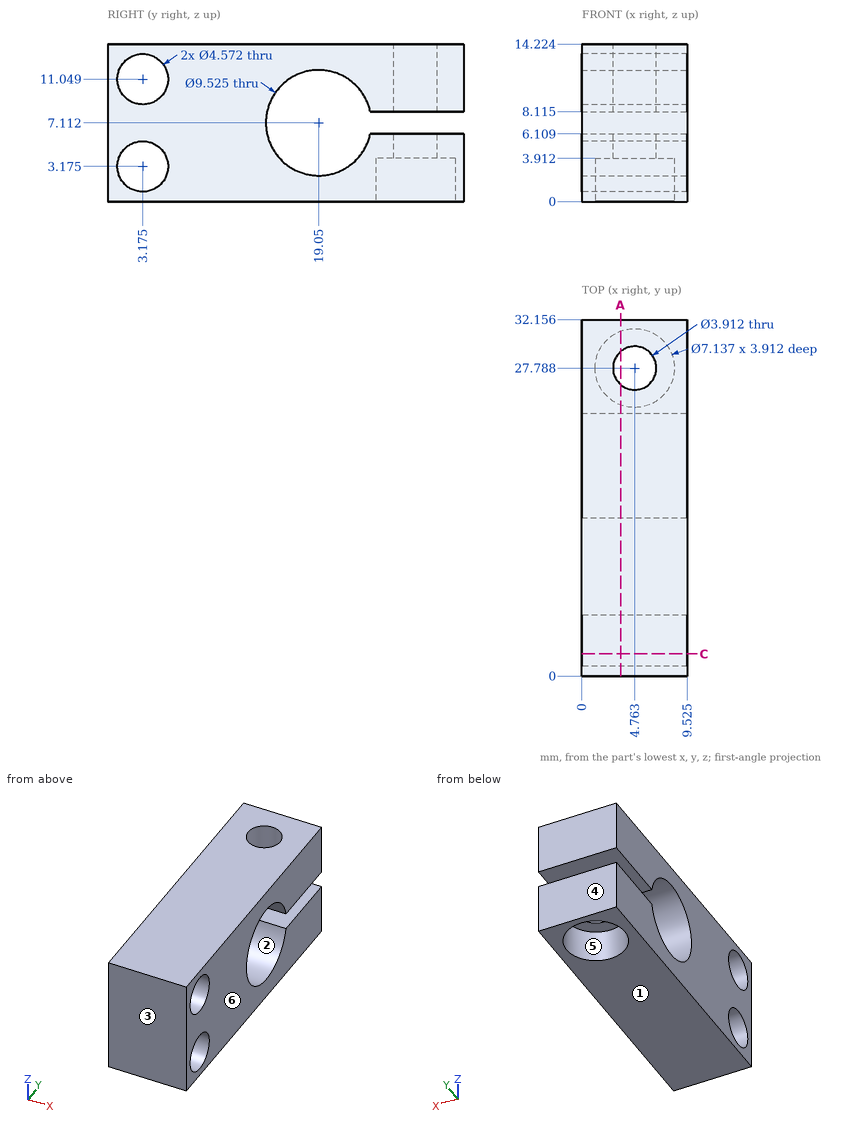
Source: three-view drawing plus pictorial views. Frame: mm from the lowest corner of the part. A direction names the side the tool comes from. Give positions to 0.01 mm unless a question says otherwise; leave off trailing zeros. Order: outer loops, then holes, each group sorted by start corner. A loop starts at its lowest first (then second) coordinate and runs counter-clockwise, first axis right, second up. Notation, with made-up numbers: (83.25, 38) - (105.25, 38) arc R22 cw to (105.25, 68) - close; hole circle Ø7 at (-7.5, -17.5). An arc over 180 degrees is marked (long way). Answer as a JSON object with one key per item and string values. Group by question number.
Q1. First-contact query: pin 1 Ø3.5 at (x, y) = (4.5, 27) entering from -Z. Flat tip, straight axial feed; report the tip coordinate or a pass-through.
Q2. Cut plane A-A, the plane x = 3.5. Count the separate pieces of the cut face and the enclosed holes in it.
Q3. Line query: probe 1 along Z at (x, y) = (7.5, 25) (1 decimal); probe 2 along Y at (x, z) = (3.5, 9.25) (1 decimal); probe 3 along Y at (x, z) = (6.25, 3.25) (1 decimal). Output: solid intervals per line, ascending.
Q4. Mould query, pull axis Y, two halves, no side actions, for the marked faces 1, 2, 3 and 4. Classes: pulls with the +Y half, pulls with the -Y half, needs draft (parallel to the pull), parting line crosses it, or undercut.
Q5. Cut plane C-C, the plane y = 2. Output: boundary loops of the cut face in (x, z) (1 decimal).
Q6. Set-up query: the marked faces 5 and 6. Return all of +Z, -Z, +X, -X, +Y, -Y with unobstructed straight access to the full face (end or side cutting, diameter ignored); none if empty.
Results:
{
 "1": {"pin 1": "z = 3.91"},
 "2": {"separate pieces": "3", "enclosed holes": "2"},
 "3": {"probe 1": "0 to 6.1, 8.1 to 14.2", "probe 2": "0 to 1.8, 4.6 to 14.8, 23.3 to 26.3, 29.3 to 32.2", "probe 3": "0 to 0.9, 5.5 to 16.3, 21.8 to 24.5, 31 to 32.2"},
 "4": {"face 1": "needs draft", "face 2": "undercut", "face 3": "pulls with the -Y half", "face 4": "pulls with the +Y half"},
 "5": {"outline": "(0, 0) - (9.5, 0) - (9.5, 1.2) - (0, 1.2) - close; (0, 5.1) - (9.5, 5.1) - (9.5, 9.1) - (0, 9.1) - close; (0, 13) - (9.5, 13) - (9.5, 14.2) - (0, 14.2) - close"},
 "6": {"face 5": "-Z", "face 6": "+Z, -Z, +X, +Y, -Y"}
}
